```python
from build123d import *

# Parameters (mm, degrees)
ESQUISSE1_R      = 1.5
EXTRUSION1_DEPTH = 5
ESQUISSE2_R      = 2.5
EXTRUSION2_DEPTH = 2


with BuildPart() as part:
    # Esquisse1 → Extrusion1 (new body)
    with BuildSketch(Plane.XY):
        with BuildLine():
            Line((-13.964240044, -1), (-2.828427125, -1))
            ThreePointArc((-2.828427125, -1), (0, 3), (2.828427125, -1))
            Line((2.828427125, -1), (13.964240044, -1))
            ThreePointArc((13.964240044, -1), (0, 14), (-13.964240044, -1))
        make_face()
        with Locations((-7.071067812, 7.071067812)):
            Circle(ESQUISSE1_R, mode=Mode.SUBTRACT)
        with Locations((7.071067812, 7.071067812)):
            Circle(ESQUISSE1_R, mode=Mode.SUBTRACT)
    extrude(amount=EXTRUSION1_DEPTH)

    # Esquisse2 → Extrusion2 (cut)
    with BuildSketch(Plane.XY.offset(5)):
        with Locations((-7.071067812, 7.071067812)):
            Circle(ESQUISSE2_R)
        with Locations((7.071067812, 7.071067812)):
            Circle(ESQUISSE2_R)
    extrude(amount=-EXTRUSION2_DEPTH, mode=Mode.SUBTRACT)


solid = part.part
```
The model under review builds one solid part; all positions refer to its coordinate system, in mm. A direction names the side the tool comes from. Coordinates: 2 decimals unless noted, no trailing zeros. Write each loop counter-clockwise with the first axis right and the second up, starting at its lowest first coordinate (ties: lowest second). Pieces come first, ordered by that corner, then holes. Notation, with made-up numbers: (42, -5.5) - (52, -5.5) arc R11 ccw to (52, 1.5) - close; hole circle Ø9 at (81.5, -32). An arc over 180 degrees is marked (long way). Write item = value, one per line.
(1) For line 1 (X direction, y = 5, z = 4.3); line 2 (X direction, y = 0, z = 1.95); line 3 (X direction, y = 7, z = 2.9), list the stretches that pass through material, from the lowest coordinate up. Write a range as [from, to].
Result sheet:
line_1 = [-13.08, -8.47], [-5.67, 5.67], [8.47, 13.08]
line_2 = [-14, -3], [3, 14]
line_3 = [-12.12, -8.57], [-5.57, 5.57], [8.57, 12.12]
(2) Consider section A-A, the plane y = 1. Give the boundary of the cut face in (x, z), then the cut area to 3 significant figures.
Result sheet:
outline = (-13.96, 0) - (-2.83, 0) - (-2.83, 5) - (-13.96, 5) - close; (2.83, 0) - (13.96, 0) - (13.96, 5) - (2.83, 5) - close
area = 111 mm^2
(3) For P1, Ø1.5, axis at x = -9, z = 2, coming from the +Y side; P2, Ø1.5, axis at x = -2.5, z = 2.5, coming from the +Y side, all flat-tipped, find the tip position at first contact; note any pin that passes through.
Result sheet:
P1 = 11.31
P2 = 13.89
(4) Consider section C-C, the plane z = 1.4. Give the boundary of the cut face in (x, y).
Result sheet:
outline = (-13.96, -1) - (-2.83, -1) arc R3 cw (long way) to (2.83, -1) - (13.96, -1) arc R14 ccw (long way) to start; hole circle Ø3 at (-7.07, 7.07); hole circle Ø3 at (7.07, 7.07)
(5) Consider section D-D, the plane x = 5.25. Give the boundary of the cut face in (y, z), then the cut area to 3 significant figures.
Result sheet:
outline = (-1, 0) - (12.98, 0) - (12.98, 5) - (8.78, 5) - (8.78, 3) - (5.36, 3) - (5.36, 5) - (-1, 5) - close
area = 63.0 mm^2
(6) Machinability: for faces 1 (the face through (-5, 7, 3)), 2 (the face through (-5.685, 6.497, 1.479)), which of the approach directions +Z, -Z, +X, -X, +Y, -Y give a long, thin tool a straight path to every point of the face, cutting with its end or side? Answer none if there is none.
Result sheet:
face_1 = +Z
face_2 = +Z, -Z
(7) Mouldability with a two-part tool opening along Y and no side actions: class faces 3 (the face through (4.573, 7.181, 4.014)), 4 (the face through (-9.57, 7.18, 4.01)), 5 (the face through (8, -1, 2)), 6 (the face through (0, 5, 5)) as pulls with the +Y half, pulls with the -Y half, needs draft (parallel to the pull), parting line crosses it, or undercut.
Result sheet:
face_3 = undercut
face_4 = undercut
face_5 = pulls with the -Y half
face_6 = needs draft
(8) Consider section B-B, the plane x = 0. Give the boundary of the cut face in (y, z).
Result sheet:
outline = (3, 0) - (14, 0) - (14, 5) - (3, 5) - close
